Check sheet for the modelled part. Datum: model origin and axes. Units: mm. Face numbers are marked on the shaded views. Round coordinates to 2 decimals unless told otherwise and drop trailing zeros. Order: outer loops, then holes, each group sorted by start corner. A loop starts at its lowest first (then second) coordinate and runs counter-clockwise, first axis right, second up.
Q1. Mould release check, pull along Y, two halves, no side actions. Record for the marked faces 1, 2 and 3: +Y half, -Y half, draft (parallel to the pull), parting line (faces both ways), or undercut.
Q2. Cross-section at A-A on z = 0. Record the cut outline in (x, y).
Q3. Scan lines: probe 1 along Z at (x, y) = (7.25, 0); probe 2 along Y at (x, z) = (17.5, -8); probe 3 along X at (y, z) = (31.5, 14.5). Record each from-to range of solid material in increasing order.
Q4. Depth check by flat-ended pin: P1, Ø1.5, axis at x = 8, z = -15, coming from the -Y side; P2, Ø2, axis at x = 5, z = -28, coming from the -Y side; P3, Ø10, axis at x = 12, z = -21, coming from the +Y side. Enter the tip coordinate at first touch or a pass-through.
Q5. Cross-section at D-D on x = 1.75. Record the cut outline in (y, z).
Q6. Cross-section at C-C on x = 9.75. Record the cut outline in (y, z), then the cut area to 3 significant figures.
from build123d import *

# Parameters (mm, degrees)
F0_R     = 41.093721
F1_DEPTH = 19
F2_R     = 6.759798
F3_R     = 8.635664
F4_DEPTH = 34.1


with BuildPart() as f1:
    # F0 (on Right) → F1 (new body)
    with BuildSketch(Plane.YZ):
        Circle(F0_R)
    extrude(amount=F1_DEPTH)

    # F2
    f2_edges = [f1.edges().sort_by_distance(p)[0] for p in [
        (19, -41.093721, 0),
        (0, -41.093721, 0),
    ]]
    fillet(f2_edges, radius=F2_R)

    # F3 (on Right) → F4 (cut, symmetric)
    with BuildSketch(Plane.YZ):
        Circle(F3_R)
    extrude(amount=F4_DEPTH, both=True, mode=Mode.SUBTRACT)


solid = f1.part
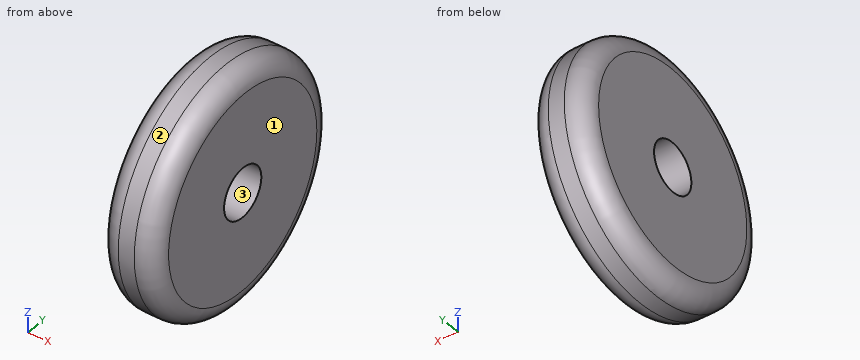
Results found:
1. face 1: draft
1. face 2: parting line
1. face 3: undercut
2. outline: (0, -34.33) arc R6.76 ccw to (6.76, -41.09) - (12.24, -41.09) arc R6.76 ccw to (19, -34.33) - (19, -8.64) - (0, -8.64) - close; (0, 8.64) - (19, 8.64) - (19, 34.33) arc R6.76 ccw to (12.24, 41.09) - (6.76, 41.09) arc R6.76 ccw to (0, 34.33) - close
3. probe 1: z = -41.09 to -8.64, 8.64 to 41.09
3. probe 2: y = -37.74 to -3.25, 3.25 to 37.74
3. probe 3: x = 0.01 to 18.99
4. P1: stops at y = -38.54
4. P2: stops at y = -30.73
4. P3: stops at y = 37.85
5. outline: circle Ø77.74 at (0, 0); hole circle Ø17.27 at (0, 0)
6. outline: circle Ø82.19 at (0, 0); hole circle Ø17.27 at (0, 0)
6. area: 5,070 mm2
